Design review of the part built by this model. Coordinates are the model's own, in mm. A direction names the side the tool comes from. Round coordinates to 2 decimals unless told otherwise and drop trailing zeros. Write each loop counter-clockwise with the first axis right and the second up, starting at its lowest first coordinate (ties: lowest second). Pieces come first, ordered by that corner, then holes. Notation, with made-up numbers: (77, 17.5) - (109, 17.5) arc R6 ccw to (109, 21.5) - close; hole circle Ø11 at (-8.5, 64.5). An arc over 180 degrees is marked (long way). Use one line per item in the form item = value.
```python
from build123d import *

# Parameters (mm, degrees)
ESQUISSE1_W               = 150
ESQUISSE1_H               = 70
BOSS_EXTRU_1_DEPTH        = 3
ESQUISSE2_W               = 9
ESQUISSE2_H               = 12
ESQUISSE2_R               = 2.25
BOSS_EXTRU_2_DEPTH        = 10
SYM_TRIE2_COPY_1_SKETCH_W = 9
SYM_TRIE2_COPY_1_SKETCH_H = 12
SYM_TRIE2_COPY_1_SKETCH_R = 2.25
SYM_TRIE2_COPY_1_DEPTH    = 10
ESQUISSE3_W               = 10
ESQUISSE3_H               = 6
ESQUISSE3_R               = 2.25
BOSS_EXTRU_3_DEPTH        = 10
SYM_TRIE4_COPY_1_SKETCH_W = 10
SYM_TRIE4_COPY_1_SKETCH_H = 6
SYM_TRIE4_COPY_1_SKETCH_R = 2.25
SYM_TRIE4_COPY_1_DEPTH    = 10
BOSS_EXTRU_4_DEPTH        = 10
BOSS_EXTRU_4_DEPTH_BACK   = 30
CONG_1_R                  = 5
CONG_2_R                  = 4
ENL_V_MAT_EXTRU_1_REACH   = 169.881
ESQUISSE5_R               = 4
ESQUISSE6_W               = 23.3
ESQUISSE6_H               = 6
ESQUISSE6_W_2             = 6.3
ESQUISSE6_H_2             = 45
BOSS_EXTRU_5_DEPTH        = 6
CHANFREIN1_SIZE           = 1.7
ESQUISSE7_W               = 15
ESQUISSE7_H               = 6
ESQUISSE7_W_2             = 32.4
BOSS_EXTRU_6_DEPTH        = 6
CHANFREIN2_SIZE           = 5
CHANFREIN3_SIZE           = 25
ESQUISSE8_R               = 5
ENL_V_MAT_EXTRU_2_DEPTH   = 168.406690517
ESQUISSE9_R               = 7.5
ENL_V_MAT_EXTRU_3_DEPTH   = 168.406690517
ESQUISSE10_W              = 10
ESQUISSE10_H              = 1
ESQUISSE10_H_2            = 3
BOSS_EXTRU_7_DEPTH        = 10


with BuildPart() as part:
    # Esquisse1 → Boss.-Extru.1 (new body)
    with BuildSketch(Plane.XY):
        with Locations((75, 35)):
            Rectangle(ESQUISSE1_W, ESQUISSE1_H)
    extrude(amount=BOSS_EXTRU_1_DEPTH)

    # Esquisse2 → Boss.-Extru.2 (add)
    with BuildSketch(Plane.XY.offset(3)):
        with Locations((4.5, 64)):
            Rectangle(ESQUISSE2_W, ESQUISSE2_H)
        with Locations((4, 63.9)):
            Circle(ESQUISSE2_R, mode=Mode.SUBTRACT)
    boss_extru_2 = extrude(amount=BOSS_EXTRU_2_DEPTH)

    # Symétrie1: Boss.-Extru.2 across plane
    add(boss_extru_2.mirror(Plane.ZY.offset(-25.2)))

    # Symétrie2: Boss.-Extru.2 across plane
    add(boss_extru_2.mirror(Plane(origin=(0, 35, 0), x_dir=(0, 0, 1), z_dir=(0, -1, 0))))

    # Symétrie2 copy 1 sketch → Symétrie2 copy 1 (add)
    with BuildSketch(Plane(origin=(50.4, 70, 3), x_dir=(-1, 0, 0), z_dir=(0, 0, 1))):
        with Locations((4.5, 64)):
            Rectangle(SYM_TRIE2_COPY_1_SKETCH_W, SYM_TRIE2_COPY_1_SKETCH_H)
        with Locations((4, 63.9)):
            Circle(SYM_TRIE2_COPY_1_SKETCH_R, mode=Mode.SUBTRACT)
    extrude(amount=SYM_TRIE2_COPY_1_DEPTH)

    # Esquisse3 → Boss.-Extru.3 (add)
    with BuildSketch(Plane.XY.offset(3)):
        with Locations((70.4, 67)):
            Rectangle(ESQUISSE3_W, ESQUISSE3_H)
        with Locations((68.85, 66.55)):
            Circle(ESQUISSE3_R, mode=Mode.SUBTRACT)
    boss_extru_3 = extrude(amount=BOSS_EXTRU_3_DEPTH)

    # Symétrie3: Boss.-Extru.3 across plane
    add(boss_extru_3.mirror(Plane.ZY.offset(-87.05)))

    # Symétrie4: Boss.-Extru.3 across plane
    add(boss_extru_3.mirror(Plane.ZX.offset(48.35)))

    # Symétrie4 copy 1 sketch → Symétrie4 copy 1 (add)
    with BuildSketch(Plane(origin=(174.1, 96.7, 3), x_dir=(-1, 0, 0), z_dir=(0, 0, 1))):
        with Locations((70.4, 67)):
            Rectangle(SYM_TRIE4_COPY_1_SKETCH_W, SYM_TRIE4_COPY_1_SKETCH_H)
        with Locations((68.85, 66.55)):
            Circle(SYM_TRIE4_COPY_1_SKETCH_R, mode=Mode.SUBTRACT)
    extrude(amount=SYM_TRIE4_COPY_1_DEPTH)

    # Esquisse4 → Boss.-Extru.4 (add, two sides: drawn at the far end of the back side and taken through both)
    with BuildSketch(Plane(origin=(0, 35, 0), x_dir=(-1, 0, 0), z_dir=(0, -1, 0)).offset(-BOSS_EXTRU_4_DEPTH_BACK)):
        Polygon((-150, -3), (-150, -28), (-148, -28), (-132.5, -12.5), (-117, -28), (-115, -28), (-115, -3), align=None)
    extrude(amount=BOSS_EXTRU_4_DEPTH + BOSS_EXTRU_4_DEPTH_BACK)

    # Congé1
    cong_1_edges = [part.edges().sort_by_distance(p)[0] for p in [
        (132.5, 45, 12.5),
    ]]
    fillet(cong_1_edges, radius=CONG_1_R)

    # Congé2
    cong_2_edges = [part.edges().sort_by_distance(p)[0] for p in [
        (117, 45, 28),
        (148, 45, 28),
    ]]
    fillet(cong_2_edges, radius=CONG_2_R)

    # Enlèv. mat.-Extru.1: up to this face of the body (flat: up to its plane)
    enl_v_mat_extru_1_end = Plane(part.part.faces().sort_by_distance((115, 45, 15.5))[0])
    # Esquisse5 → Enlèv. mat.-Extru.1 (cut, up to the picked face)
    with BuildSketch(Plane(origin=(150, 0, 0), x_dir=(0, 0, -1), z_dir=(1, 0, 0)), mode=Mode.PRIVATE) as enl_v_mat_extru_1_sk1:
        with Locations((-13, 52)):
            Circle(ESQUISSE5_R)
    enl_v_mat_extru_1_tool1 = split(extrude(enl_v_mat_extru_1_sk1.sketch, amount=-ENL_V_MAT_EXTRU_1_REACH, mode=Mode.PRIVATE), bisect_by=enl_v_mat_extru_1_end, keep=Keep.BOTH, mode=Mode.PRIVATE)
    # Esquisse5 → Enlèv. mat.-Extru.1 (cut, up to the picked face)
    with BuildSketch(Plane(origin=(150, 0, 0), x_dir=(0, 0, -1), z_dir=(1, 0, 0)), mode=Mode.PRIVATE) as enl_v_mat_extru_1_sk2:
        with Locations((-13, 38)):
            Circle(ESQUISSE5_R)
    enl_v_mat_extru_1_tool2 = split(extrude(enl_v_mat_extru_1_sk2.sketch, amount=-ENL_V_MAT_EXTRU_1_REACH, mode=Mode.PRIVATE), bisect_by=enl_v_mat_extru_1_end, keep=Keep.BOTH, mode=Mode.PRIVATE)
    add(enl_v_mat_extru_1_tool1.solids().sort_by(Axis((150, 52, 13), (-1, 0, 0)))[0], mode=Mode.SUBTRACT)
    add(enl_v_mat_extru_1_tool2.solids().sort_by(Axis((150, 38, 13), (-1, 0, 0)))[0], mode=Mode.SUBTRACT)

    # Esquisse6 → Boss.-Extru.5 (add)
    with BuildSketch(Plane.XY.offset(3)):
        with Locations((87.05, 67)):
            Rectangle(ESQUISSE6_W, ESQUISSE6_H)
        with Locations((87.05, 29.7)):
            Rectangle(ESQUISSE6_W, ESQUISSE6_H)
        with Locations((111.85, 47.5)):
            Rectangle(ESQUISSE6_W_2, ESQUISSE6_H_2)
    extrude(amount=BOSS_EXTRU_5_DEPTH)

    # Chanfrein1
    chanfrein1_edges = [part.edges().sort_by_distance(p)[0] for p in [
        (108.7, 25, 6),
    ]]
    chamfer(chanfrein1_edges, length=CHANFREIN1_SIZE - 0.0001)  # a hair under: the kernel refuses the full size

    # Esquisse7 → Boss.-Extru.6 (add)
    with BuildSketch(Plane.XY.offset(3)):
        with Locations((57.9, 67)):
            Rectangle(ESQUISSE7_W, ESQUISSE7_H)
        with Locations((25.2, 67)):
            Rectangle(ESQUISSE7_W_2, ESQUISSE7_H)
    extrude(amount=BOSS_EXTRU_6_DEPTH)

    # Chanfrein2
    chanfrein2_edges = [part.edges().sort_by_distance(p)[0] for p in [
        (150, 70, 1.5),
    ]]
    chamfer(chanfrein2_edges, length=CHANFREIN2_SIZE)

    # Chanfrein3
    chanfrein3_edges = [part.edges().sort_by_distance(p)[0] for p in [
        (150, 0, 1.5),
    ]]
    chamfer(chanfrein3_edges, length=CHANFREIN3_SIZE)

    # Esquisse8 → Enlèv. mat.-Extru.2 (cut, through all)
    with BuildSketch(Plane.XY.offset(3)):
        with Locations((56.4, 58)):
            Circle(ESQUISSE8_R)
    extrude(amount=-ENL_V_MAT_EXTRU_2_DEPTH, mode=Mode.SUBTRACT)

    # Esquisse9 → Enlèv. mat.-Extru.3 (cut, through all)
    with BuildSketch(Plane.XY.offset(3)):
        with Locations((110, 11.7)):
            Circle(ESQUISSE9_R)
    extrude(amount=-ENL_V_MAT_EXTRU_3_DEPTH, mode=Mode.SUBTRACT)

    # Esquisse10 → Boss.-Extru.7 (add)
    with BuildSketch(Plane.XY.offset(3)):
        with Locations((70.4, 63.5)):
            Rectangle(ESQUISSE10_W, ESQUISSE10_H)
        with Locations((103.7, 62.5)):
            Rectangle(ESQUISSE10_W, ESQUISSE10_H_2)
        with Locations((103.7, 34.2)):
            Rectangle(ESQUISSE10_W, ESQUISSE10_H_2)
    extrude(amount=BOSS_EXTRU_7_DEPTH)


solid = part.part
```
Q1. For P1, Ø3, axis at y = 6, z = 9, coming from the +X side; P2, Ø11, axis at y = 8.5, z = 7.5, coming from the +X side; P3, Ø2.5, axis at x = 6, y = 9, coming from the +Z side, all flat-tipped, find the tip position at first contact; note any pin that passes through.
Calculated:
P1 = 50.4
P2 = 136.66
P3 = 13
Q2. Draft analysis for pull direction Z (two halves, no side actions). For faces 4 (the flat face through (70, 63, 8)), 5 (the flat face through (105, 67, 3)), 6 (the cylindrical face through (132.745, 39.201, 9.185)), state which applies: released by +Z, released by -Z, zero draft, split by the parting line, or undercut.
Calculated:
face_4 = zero draft
face_5 = released by +Z
face_6 = undercut
Q3. We need section C-C on x = 127. Write out the cut boundary in (y, z).
Calculated:
outline = (2, 0) - (70, 0) - (70, 3) - (65, 3) - (65, 18) - (25, 18) - (25, 3) - (2, 3) - close; hole circle Ø8 at (38, 13); hole circle Ø8 at (52, 13)
Q4. We need section D-D on y = 30.15. Write out the cut boundary in (x, z).
Calculated:
outline = (0, 0) - (150, 0) - (150, 28) - (149.66, 28) arc R4 ccw to (146.83, 26.83) - (136.04, 16.04) arc R5 cw to (128.96, 16.04) - (118.17, 26.83) arc R4 ccw to (115.34, 28) - (115, 28) - (115, 9) - (108.7, 9) - (108.7, 13) - (107.5, 13) - (107.5, 3) - (103, 3) - (103, 13) - (98.7, 13) - (98.7, 9) - (75.4, 9) - (75.4, 13) - (71.1, 13) - (71.1, 3) - (66.6, 3) - (66.6, 13) - (65.4, 13) - (65.4, 3) - (0, 3) - close
Q5. We need section B-B on x = 56.4. Write out the cut boundary in (y, z).
Calculated:
outline = (0, 0) - (53, 0) - (53, 3) - (0, 3) - close; (63, 0) - (70, 0) - (70, 9) - (64, 9) - (64, 3) - (63, 3) - close
Q6. Machinability: for faces 1 (the flat face through (133, 65, 13)), 2 (the cylindrical face through (46.69, 66.13, 7.93)), 3 (the flat face through (58, 64, 6)), which of the approach directions +Z, -Z, +X, -X, +Y, -Y give a long, thin tool a straight path to every point of the face, cutting with its end or side? Answer none if there is none.
Calculated:
face_1 = +Z, +X, +Y
face_2 = +Z
face_3 = +Z, -Y
Q7. We need section A-A on z = 19.5. Write out the cut boundary in (x, y).
Calculated:
outline = (115, 25) - (125.5, 25) - (125.5, 65) - (115, 65) - close; (139.5, 25) - (150, 25) - (150, 65) - (139.5, 65) - close
Q8. To check wall thickness, follow line 1 along Y through (x, z) = (4, 5.75); line 2 along Y through (x, z) = (68.85, 5.5); line 3 along X through (y, z) = (60, 10.25). State the ranges of each line that lie inside material, in increasing order. Write a range as from..to.
Calculated:
line_1 = 0..3.85, 8.35..12, 58..61.65, 66.15..70
line_2 = 26.7..27.9, 32.4..32.7, 63..64.3, 68.8..70
line_3 = 0..9, 41.4..50.4, 115..150
